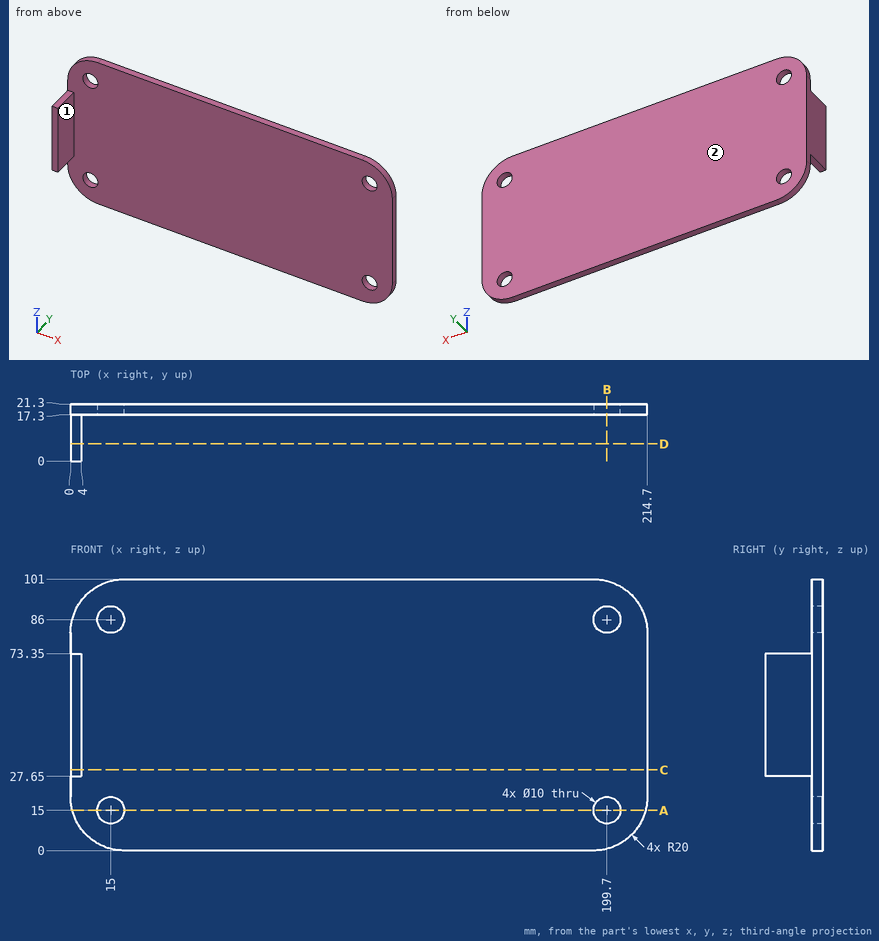
Answer from the drawing. Dimensions are ordinates in mm from the lowest x, y and z of the part. A direction names the side the tool comes from. Give positions to 0.01 mm unless a question says otherwise; leave off trailing zeros. Order: outer loops, then holes, each group sorted by start corner. A loop starts at its lowest first (then second) coordinate and runs counter-clockwise, first axis right, second up.
(1) Given pin 1 (6 mm diameter, centred on x = 154.5, z = 65, fed in from -Y); pin 2 (5 mm diameter, centred on y = 6.5, z = 57, fed in from +X); pin 3 (9 mm diameter, centred on x = 15, z = 86, fed in from -Y); pin 4 (3 mm diameter, centred on x = 2, y = 11.5, fed in from -Z), each flat-ended and moving along its own axis, determine where each tip first touches the part or whether it passes through.
(2) For the marked faces 1 and 2, determine the directions among +Z, -Z, +X, -X, +Y, -Y from which every point of the face is accessible in a straight line to the end or side of a thin tool.
(3) Straight lines are drawn through the part: L1, parallel to Z at x = 199.7, y = 18.6; L2, parallel to X at y = 19.4, z = 86; L3, parallel to Y at x = 122, z = 49. For each, find the intervals that lie inside material, in ascending order.
(4) Find section B-B (x = 199.7). Give the vertices of the cut face in (y, z), plus the area to 3 significant figures.
(5) Find section C-C (z = 30). Give the vertices of the cut face in (x, y), plus the area to 3 significant figures.
(6) Find section A-A (z = 15). Give the vertices of the cut face in (x, y).
(7) Find section D-D (y = 6.5). Give the vertices of the cut face in (x, z).
Result sheet:
1. pin 1: stops at y = 17.3
1. pin 2: stops at x = 4
1. pin 3: passes through
1. pin 4: stops at z = 27.65
2. face 1: +Z, -Z, +X, -Y
2. face 2: +Z, -Z, +X, -X, +Y
3. L1: z = 0.64 to 10, 20 to 81, 91 to 100.36
3. L2: x = 0.64 to 10, 20 to 194.7, 204.7 to 214.06
3. L3: y = 17.3 to 21.3
4. outline: (17.3, 0.64) - (21.3, 0.64) - (21.3, 10) - (17.3, 10) - close; (17.3, 20) - (21.3, 20) - (21.3, 81) - (17.3, 81) - close; (17.3, 91) - (21.3, 91) - (21.3, 100.36) - (17.3, 100.36) - close
4. area: 319 mm2
5. outline: (0, 0) - (4, 0) - (4, 17.3) - (214.7, 17.3) - (214.7, 21.3) - (0, 21.3) - close
5. area: 928 mm2
6. outline: (0.64, 17.3) - (10, 17.3) - (10, 21.3) - (0.64, 21.3) - close; (20, 17.3) - (194.7, 17.3) - (194.7, 21.3) - (20, 21.3) - close; (204.7, 17.3) - (214.06, 17.3) - (214.06, 21.3) - (204.7, 21.3) - close
7. outline: (0, 27.65) - (4, 27.65) - (4, 73.35) - (0, 73.35) - close
